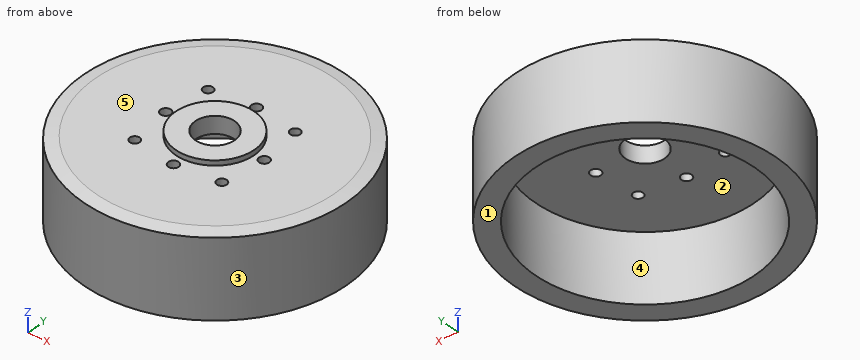
from build123d import *

# Parameters (mm, degrees)
SKETCH3_R           = 53.4
BOSS_EXTRUDE1_DEPTH = 38.5
SKETCH4_R           = 8
CUT_EXTRUDE1_DEPTH  = 85.766561804
SKETCH5_R           = 2
CUT_EXTRUDE2_DEPTH  = 20
BOSS_EXTRUDE3_START = 2
SKETCH6_R           = 16
SKETCH6_R_2         = 8
BOSS_EXTRUDE3_DEPTH = 2
SKETCH7_R           = 2.1
CUT_EXTRUDE3_DEPTH  = 20
SKETCH8_R           = 2.5
CUT_EXTRUDE4_DEPTH  = 20
CHAMFER1_SIZE       = 1
CHAMFER1_SIZE2      = 5
CUT_EXTRUDE5_START  = -6
SKETCH9_R           = 53.4
CUT_EXTRUDE5_DEPTH  = 6
SKETCH10_R          = 44.75
CUT_EXTRUDE6_DEPTH  = 27.6


with BuildPart() as part:
    # Sketch3 → Boss-Extrude1 (new body)
    with BuildSketch(Plane.XY):
        Circle(SKETCH3_R)
    extrude(amount=-BOSS_EXTRUDE1_DEPTH)

    # Sketch4 → Cut-Extrude1 (cut, through all)
    with BuildSketch(Plane.XY):
        Circle(SKETCH4_R)
    extrude(amount=-CUT_EXTRUDE1_DEPTH, mode=Mode.SUBTRACT)

    # Sketch5 → Cut-Extrude2 (cut)
    with BuildSketch(Plane.XY):
        with Locations((-17.67766953, 17.67766953)):
            Circle(SKETCH5_R)
        with Locations((17.67766953, 17.67766953)):
            Circle(SKETCH5_R)
        with Locations((-17.67766953, -17.67766953)):
            Circle(SKETCH5_R)
        with Locations((17.67766953, -17.67766953)):
            Circle(SKETCH5_R)
    extrude(amount=-CUT_EXTRUDE2_DEPTH, mode=Mode.SUBTRACT)

    # Sketch6 → Boss-Extrude3 (add)
    with BuildSketch(Plane.XY.offset(BOSS_EXTRUDE3_START)):
        Circle(SKETCH6_R)
        Circle(SKETCH6_R_2, mode=Mode.SUBTRACT)
    extrude(amount=-BOSS_EXTRUDE3_DEPTH)

    # Sketch7 → Cut-Extrude3 (cut)
    with BuildSketch(Plane.XY):
        with Locations((0, 20)):
            Circle(SKETCH7_R)
        with Locations((20, 0)):
            Circle(SKETCH7_R)
        with Locations((-20, 0)):
            Circle(SKETCH7_R)
        with Locations((0, -20)):
            Circle(SKETCH7_R)
    extrude(amount=-CUT_EXTRUDE3_DEPTH, mode=Mode.SUBTRACT)

    # Sketch8 → Cut-Extrude4 (cut)
    with BuildSketch(Plane(origin=(0, 0, -38.5), x_dir=(-1, 0, 0), z_dir=(0, 0, -1))):
        with Locations((0, 30)):
            Circle(SKETCH8_R)
        with Locations((30, 0)):
            Circle(SKETCH8_R)
        with Locations((0, -30)):
            Circle(SKETCH8_R)
        with Locations((-30, 0)):
            Circle(SKETCH8_R)
    extrude(amount=-CUT_EXTRUDE4_DEPTH, mode=Mode.SUBTRACT)

    # Chamfer1
    chamfer1_edges = [part.edges().sort_by_distance(p)[0] for p in [
        (-53.4, 0, 0),
    ]]
    chamfer1_side = [part.faces().sort_by_distance(p)[0] for p in [
        (-53.4, 0, -19.25),
    ]]
    chamfer(chamfer1_edges, length=CHAMFER1_SIZE, length2=CHAMFER1_SIZE2, reference=chamfer1_side[0])

    # Sketch9 → Cut-Extrude5 (cut)
    with BuildSketch(Plane(origin=(0, 0, -38.5), x_dir=(-1, 0, 0), z_dir=(0, 0, -1)).offset(CUT_EXTRUDE5_START)):
        with Locations(Location((0, 0, 0), (0, 0, 180))):
            Circle(SKETCH9_R)
    extrude(amount=CUT_EXTRUDE5_DEPTH, mode=Mode.SUBTRACT)

    # Sketch10 → Cut-Extrude6 (cut)
    with BuildSketch(Plane(origin=(0, 0, -32.5), x_dir=(-1, 0, 0), z_dir=(0, 0, -1))):
        Circle(SKETCH10_R)
    extrude(amount=-CUT_EXTRUDE6_DEPTH, mode=Mode.SUBTRACT)


solid = part.part
Read the model definition and answer for the solid it produces. Units are mm, in the model's axes. Face numbers are marked on the shaded views. A direction names the side the tool comes from. Give positions to 0.01 mm unless a question says otherwise; leave off trailing zeros. Loops run counter-clockwise (first coordinate to the right, second up) from the corner with the lowest first, then second, coordinate; pieces in that order, holes last. Notation, with made-up numbers: (-2, -12) - (54, -12) arc R8 cw to (54, -2) - close; hole circle Ø3 at (-21, 57.5). An arc over 180 degrees is marked (long way). Answer as CSV lines item,"result". Start each with the question number.
1) Which of the six approach directions +Z, -Z, +X, -X, +Y, -Y give full straight-line access (tool end or side, diameter ignored) to the marked faces 1 and 2?
2) Find section A-A (x = 0). Write down the section's boundary in (y, z), then the cut area to 3 significant figures.
3) Determine the mould class of the marked faces 3, 4 and 5 for opening direction Y: released by +Y, released by -Y, zero draft, split by the parting line, or undercut.
4) Find section B-B (z = -15). Write down the section's boundary in (x, y), then the cut area to 3 significant figures.
5) Straight lines are drawn through the part: L1, parallel to Y at x = 0, z = -2; L2, parallel to Y at x = 0, z = -22.25; L3, parallel to Z at x = 10.5, y = 42. For each, find the intervals that lie inside material, in ascending order. Write a range as from..to.
6) Each of these flat-tipped pins is pushed along its axis until it touches: pin 1 Ø3 at (y, z) = (18, -26.5) entering from -X; pin 2 Ø12 at (y, z) = (19, -7) entering from +X; pin 3 Ø8 at (x, z) = (-17.5, -13) entering from -Y. Where does it stop, or does it pass through?
Findings below:
1,face 1,"-Z, +X, -X, +Y, -Y"
1,face 2,"-Z"
2,outline,"(-53.4, -32.5) - (-44.75, -32.5) - (-44.75, -4.9) - (-22.1, -4.9) - (-22.1, 0) - (-48.4, 0) - (-53.4, -1) - close; (-17.9, -4.9) - (-8, -4.9) - (-8, 2) - (-16, 2) - (-16, 0) - (-17.9, 0) - close; (8, -4.9) - (17.9, -4.9) - (17.9, 0) - (16, 0) - (16, 2) - (8, 2) - close; (22.1, -4.9) - (44.75, -4.9) - (44.75, -32.5) - (53.4, -32.5) - (53.4, -1) - (48.4, 0) - (22.1, 0) - close"
2,area,"908 mm^2"
3,face 3,"split by the parting line"
3,face 4,"undercut"
3,face 5,"zero draft"
4,outline,"circle Ø106.8 at (0, 0); hole circle Ø89.5 at (0, 0)"
4,area,"2,670 mm^2"
5,L1,"-53.4..-22.1, -17.9..-8, 8..17.9, 22.1..53.4"
5,L2,"-53.4..-44.75, 44.75..53.4"
5,L3,"-4.9..0"
6,pin 1,"x = -50.79"
6,pin 2,"x = 51.79"
6,pin 3,"y = -51.67"
